Check sheet for the modelled part. Datum: model origin and axes. Units: mm. A direction names the side the tool comes from. Coordinates: 2 decimals unless noted, no trailing zeros. Write each loop counter-clockwise with the first axis right and the second up, starting at its lowest first coordinate (ties: lowest second). Pieces come first, ordered by that corner, then holes. Notation, with made-up numbers: (35.5, 64) -> (81.5, 64) arc R10 ccw to (81.5, 71) -> close; hole circle Ø1 at (64, 26). An arc over 180 degrees is marked (long way). One line per item, written item: value. Start each with the question number.
1) Gauge pin test, flat ends, axial feed: P1, Ø10, axis at y = 12.5, z = 22.5, coming from the +X side; P2, Ø20, axis at x = 0, y = 0, coming from the +Z side; P3, Ø1.8, axis at x = 0, y = -8, coming from the -Z side; P4, Ø6, axis at y = -6, z = 16, coming from the +X side. Record the tip position at first contact, or that the pin passes through.
2) Sectioned sample at C-C on x = -20. Enter the section's corners in (y, z), plus the area to 3 significant figures.
3) Sectioned sample at B-B on y = -8. Enter the section's corners in (x, z), plus the area to 3 significant figures.
4) Draft check along Z on faces 1 (the cylindrical face through (-3.3, -14.88, 17.32)), 2 (the flat face through (2, 5, 1.2)), 3 (the cylindrical face through (2.4, -4.5, 3.1)), 4 (the flat face through (11, -11, 30)). Enter one of: +Z half, -Z half, draft (parallel to the pull), parting line (faces both ways), or undercut.
5) Sectioned sample at D-D on z = 14. Enter the section's corners in (x, y).
6) Scan lines: line 1 along Y through (x, z) = (0, 2); line 2 along Z through (x, y) = (16, 4); line 3 along X through (y, z) = (-0.5, 29). Record each from-to range of solid material in increasing order. Write a range as [from, to].
7) Set-up check for faces 5 (the cylindrical face through (-1.445, -11.006, 0.592)), 6 (the flat face through (11, -11, 5)), 7 (the flat face through (5, -2, 5)): record each of +Z, -Z, +X, -X, +Y, -Y from which the full face is reachable in a straight line by a thin tool's end or side.
8) Sectioned sample at A-A on y = 0. Give the number of separate pieces and of enclosed holes in the cut face, plus the area to 3 significant figures.
```python
from build123d import *

# Parameters (mm, degrees)
SKETCH1_R           = 15.24
SKETCH1_R_2         = 11.1
BOSS_EXTRUDE1_DEPTH = 30
SKETCH3_R           = 25.4
SKETCH3_R_2         = 5.1
SKETCH3_R_3         = 1.5
BOSS_EXTRUDE2_DEPTH = 5
SKETCH4_R           = 25.4
SKETCH4_R_2         = 11.1
BOSS_EXTRUDE3_DEPTH = 5
SKETCH5_R           = 11.1
CUT_EXTRUDE1_DEPTH  = 1.2
SKETCH10_R          = 1.25


with BuildPart() as part:
    # Sketch1 → Boss-Extrude1 (new body)
    with BuildSketch(Plane.XY):
        Circle(SKETCH1_R)
        Circle(SKETCH1_R_2, mode=Mode.SUBTRACT)
    extrude(amount=BOSS_EXTRUDE1_DEPTH)

    # Sketch3 → Boss-Extrude2 (add)
    with BuildSketch(Plane.XY):
        Circle(SKETCH3_R)
        Circle(SKETCH3_R_2, mode=Mode.SUBTRACT)
        with Locations((0, 8)):
            Circle(SKETCH3_R_3, mode=Mode.SUBTRACT)
        with Locations((8, 0)):
            Circle(SKETCH3_R_3, mode=Mode.SUBTRACT)
        with Locations((0, -8)):
            Circle(SKETCH3_R_3, mode=Mode.SUBTRACT)
        with Locations((-8, 0)):
            Circle(SKETCH3_R_3, mode=Mode.SUBTRACT)
    extrude(amount=BOSS_EXTRUDE2_DEPTH)

    # Sketch4 → Boss-Extrude3 (add)
    with BuildSketch(Plane.XY.offset(30)):
        Circle(SKETCH4_R)
        Circle(SKETCH4_R_2, mode=Mode.SUBTRACT)
    extrude(amount=BOSS_EXTRUDE3_DEPTH)

    # Sketch5 → Cut-Extrude1 (cut)
    with BuildSketch(Plane(origin=(0, 0, 0), x_dir=(-1, 0, 0), z_dir=(0, 0, -1))):
        with Locations(Location((0, 0, 0), (0, 0, 180))):
            Circle(SKETCH5_R)
    extrude(amount=-CUT_EXTRUDE1_DEPTH, mode=Mode.SUBTRACT)

    # Sweep3: sweep along a path in Sketch14
    with BuildLine(Plane(origin=(0, 0, 0), x_dir=(0, 0, -1), z_dir=(1, 0, 0))) as sweep3_path:
        Line((-5, 22.86), (-12.988321423, 13.120638521))
    # Sketch10 → Sweep3 (sweep)
    with BuildSketch(Plane.XY.offset(5)):
        with Locations((0, 22.86)):
            Circle(SKETCH10_R)
    sweep(path=sweep3_path.line)


solid = part.part
```
Answers:
1. P1: stops at x = 13.27
1. P2: stops at z = 5
1. P3: passes through
1. P4: stops at x = 14.94
2. outline: (-15.66, 0) -> (15.66, 0) -> (15.66, 5) -> (-15.66, 5) -> close; (-15.66, 30) -> (15.66, 30) -> (15.66, 35) -> (-15.66, 35) -> close
2. area: 313 mm2
3. outline: (-24.11, 0) -> (-7.69, 0) -> (-7.69, 1.2) -> (-1.5, 1.2) -> (-1.5, 5) -> (-7.69, 5) -> (-7.69, 35) -> (-24.11, 35) -> (-24.11, 30) -> (-12.97, 30) -> (-12.97, 5) -> (-24.11, 5) -> close; (1.5, 1.2) -> (7.69, 1.2) -> (7.69, 0) -> (24.11, 0) -> (24.11, 5) -> (12.97, 5) -> (12.97, 30) -> (24.11, 30) -> (24.11, 35) -> (7.69, 35) -> (7.69, 5) -> (1.5, 5) -> close
3. area: 639 mm2
4. face 1: undercut
4. face 2: -Z half
4. face 3: draft
4. face 4: undercut
5. outline: circle Ø30.48 at (0, 0); hole circle Ø22.2 at (0, 0)
6. line 1: y = [-25.4, -9.5], [-6.5, -5.1], [5.1, 6.5], [9.5, 25.4]
6. line 2: z = [0, 5], [30, 35]
6. line 3: x = [-15.23, -11.09], [11.09, 15.23]
7. face 5: -Z
7. face 6: none
7. face 7: +Z
8. separate pieces: 4
8. enclosed holes: 0
8. area: 516 mm2
